Verification items for the finished model (mm, model axes). Face numbers are marked on the shaded views. Give positions to 0.01 mm unless a question says otherwise; leave off trailing zeros. Order: outer loops, then holes, each group sorted by start corner. A loop starts at its lowest first (then second) coordinate and runs counter-clockwise, first axis right, second up. Notation, with made-up numbers: (20.5, -19.75) - (58.5, -19.75) arc R16 ccw to (58.5, 6.25) - close; hole circle Ø4 at (65.25, 57). An arc over 180 degrees is marked (long way). Answer as a JSON object with one key per item and string values. Group by question number.
(1) Section check D-D (y = 30). Record the boundary of the cut face in (x, z) (1 decimal).
(2) Mould release check, pull along X, two halves, no side actions. Record for the marked faces 1, 2 and 3: +X half, -X half, draft (parallel to the pull), parting line (faces both ways), or undercut.
(3) Thickness scan on line 1 (X direction, y = -0.8, z = 0); line 2 (X direction, y = 35.2, z = 0); line 3 (Y direction, x = -7, z = 0.25). Record the ranges inside material, lowest first.
(4) Section check B-B (z = 0). Count the separate pieces of the cut face and the enclosed holes in it, then the cut area to 3 significant figures.
(5) Section check C-C (x = 0). Record the boundary of the cut face in (y, z).
(6) Depth check by flat-ended pin: pin 1 Ø1.1 at (x, z) = (0, 9) entering from -Y; pin 2 Ø0.5 at (x, y) = (12.5, -0.5) entering from +Z; pin 3 Ø0.5 at (x, y) = (-13.5, -0.5) entering from -Z. Enter the tip coordinate at first touch or a pass-through.
(7) Section check A-A (y = 6). Record the boundary of the cut face in (x, z) (1 decimal).
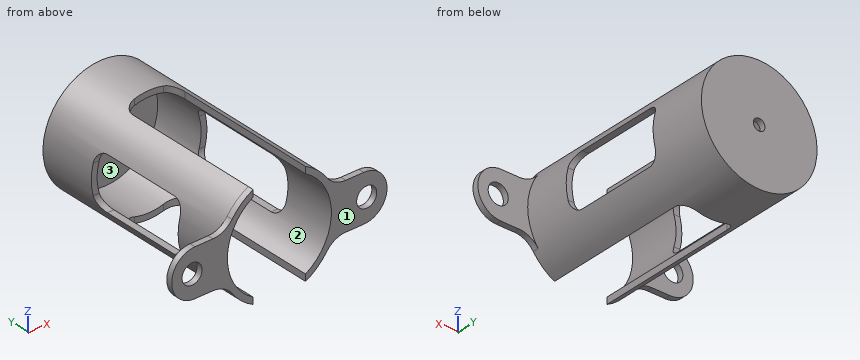
```python
from build123d import *

# Parameters (mm, degrees)
SKETCH2_R           = 9.9375
BOSS_EXTRUDE1_DEPTH = 35.384
SKETCH4_R           = 1
CUT_EXTRUDE2_DEPTH  = 39.072762817
BOSS_EXTRUDE2_START = 1
SKETCH11_R          = 8.9375
BOSS_EXTRUDE2_DEPTH = 1
SKETCH12_R          = 8.9375
CUT_EXTRUDE7_DEPTH  = 34.384
CUT_EXTRUDE8_START  = -1
CUT_EXTRUDE8_DEPTH  = 26.538
SKETCH14_W          = 9
SKETCH14_H          = 17.692
CUT_EXTRUDE9_DEPTH  = 61.852537846
FILLET3_R           = 2
FILLET4_R           = 4
CUT_EXTRUDE10_REACH = 43.146
SKETCH15_R          = 1.7272


# Read off the part's stored shape, not the designer's step: Cut-Extrude8
with BuildPart() as part:
    # Sketch2 → Boss-Extrude1 (new body)
    with BuildSketch(Plane(origin=(0, 0, 0), x_dir=(1, 0, 0), z_dir=(0, 1, 0))):
        with Locations(Location((0, 0, 0), (0, 0, 270))):
            Circle(SKETCH2_R)
    extrude(amount=BOSS_EXTRUDE1_DEPTH)

    # Sketch4 → Cut-Extrude2 (cut, through all)
    with BuildSketch(Plane(origin=(0, 35.384, 0), x_dir=(1, 0, 0), z_dir=(0, 1, 0))):
        with Locations(Location((0, 0, 0), (0, 0, 270))):
            Circle(SKETCH4_R)
    extrude(amount=-CUT_EXTRUDE2_DEPTH, mode=Mode.SUBTRACT)

    # Sketch11 → Boss-Extrude2 (add)
    with BuildSketch(Plane.XZ.offset(BOSS_EXTRUDE2_START)):
        with BuildLine():
            Line((9.096917404, 4), (18.5, 4))
            Line((18.5, 4), (18.5, -4))
            Line((18.5, -4), (9.096917404, -4))
            ThreePointArc((9.096917404, -4), (0, -9.9375), (-9.096917404, -4))
            Line((-9.096917404, -4), (-18.5, -4))
            Line((-18.5, -4), (-18.5, 4))
            Line((-18.5, 4), (-9.096917404, 4))
            ThreePointArc((-9.096917404, 4), (0, 9.9375), (9.096917404, 4))
        make_face()
        with Locations(Location((0, 0, 0), (0, 0, 270))):
            Circle(SKETCH11_R, mode=Mode.SUBTRACT)
    extrude(amount=-BOSS_EXTRUDE2_DEPTH)

    # Sketch12 → Cut-Extrude7 (cut)
    with BuildSketch(Plane.XZ):
        with Locations(Location((0, 0, 0), (0, 0, 270))):
            Circle(SKETCH12_R)
    extrude(amount=-CUT_EXTRUDE7_DEPTH, mode=Mode.SUBTRACT)

    # Cut-Extrude8 outline → Cut-Extrude8 (cut)
    with BuildSketch(Plane(origin=(0, 0, 0), x_dir=(1, 0, 0), z_dir=(0, 1, 0)).offset(CUT_EXTRUDE8_START)):
        with BuildLine():
            ThreePointArc((4.5, -7.721975541), (0, -8.9375), (-4.5, -7.721975541))
            Line((-4.5, -7.721975541), (-4.5, -8.860243013))
            ThreePointArc((-4.5, -8.860243013), (0, -9.9375), (4.5, -8.860243013))
            Line((4.5, -8.860243013), (4.5, -7.721975541))
        make_face()
        with BuildLine():
            Line((-4.5, 8.860243013), (-4.5, 7.721975541))
            ThreePointArc((-4.5, 7.721975541), (0, 8.9375), (4.5, 7.721975541))
            Line((4.5, 7.721975541), (4.5, 8.860243013))
            ThreePointArc((4.5, 8.860243013), (0, 9.9375), (-4.5, 8.860243013))
        make_face()
    extrude(amount=CUT_EXTRUDE8_DEPTH, mode=Mode.SUBTRACT)

    # Sketch14 → Cut-Extrude9 (cut, through all)
    with BuildSketch(Plane(origin=(30, 0, 0), x_dir=(0, 0, -1), z_dir=(1, 0, 0))):
        with Locations((0, 16.692)):
            Rectangle(SKETCH14_W, SKETCH14_H)
    extrude(amount=-CUT_EXTRUDE9_DEPTH, mode=Mode.SUBTRACT)

    # Fillet3
    fillet3_edges = [part.edges().sort_by_distance(p)[0] for p in [
        (4.5, 25.538, 8.291109277),
        (4.5, 25.538, -8.291109277),
        (-4.5, 25.538, -8.291109277),
        (-4.5, 25.538, 8.291109277),
        (8.291109277, 25.538, -4.5),
        (-8.291109277, 25.538, -4.5),
        (8.291109277, 7.846, -4.5),
        (-8.291109277, 7.846, -4.5),
        (-8.291109277, 7.846, 4.5),
        (8.291109277, 7.846, 4.5),
        (8.291109277, 25.538, 4.5),
        (-8.291109277, 25.538, 4.5),
    ]]
    fillet(fillet3_edges, radius=FILLET3_R)

    # Fillet4
    # the kernel refuses this fillet: 4 mm, written as the material it adds along each edge
    with BuildSketch(Plane(origin=(9.096917404, -1, -4), x_dir=(-0.4906341894667762, 0, -0.8713656477772574), z_dir=(0, 1, 0)), Plane(origin=(-9.096917404, -1, 4), x_dir=(0.49063418946677706, 0, 0.871365647777257), z_dir=(0, 1, 0))) as fillet4_piece_1:
        with BuildLine():
            CenterArc((2.349170519, -3.980589921), FILLET4_R, 95.646730554, 54.970995912)
            Line((-1.136292073, -2.018053163), (0, 0))
            ThreePointArc((0, 0), (0.977796106, -0.048221916), (1.955592212, 0))
        make_face()
    extrude(amount=1)
    with BuildSketch(Plane(origin=(9.096917404, -1, 4), x_dir=(-0.4906341894667768, 0, 0.8713656477772572), z_dir=(0, 1, 0)), Plane(origin=(-9.096917404, -1, -4), x_dir=(0.4906341894667772, 0, -0.8713656477772569), z_dir=(0, 1, 0))) as fillet4_piece_2:
        with BuildLine():
            CenterArc((2.349170519, 3.980589921), FILLET4_R, 209.382273534, 54.970995912)
            Line((-1.136292073, 2.018053163), (0, 0))
            ThreePointArc((0, 0), (0.977796106, 0.048221916), (1.955592212, 0))
        make_face()
    extrude(amount=1)
    # the kernel refuses this fillet: 4 mm, written as the material it takes off along each edge
    with BuildSketch(Plane(origin=(18.5, -11, -4), x_dir=(0, 0, 1), z_dir=(0, 1, 0)), Plane(origin=(18.5, -11, 4), x_dir=(-1, 0, 0), z_dir=(0, 1, 0))) as fillet4_2_piece_1:
        with BuildLine():
            CenterArc((FILLET4_R, -FILLET4_R), FILLET4_R, 90, 90)
            Line((0, -FILLET4_R), (0, 0))
            Line((0, 0), (FILLET4_R, 0))
        make_face()
    extrude(amount=21, mode=Mode.SUBTRACT)
    with BuildSketch(Plane(origin=(-18.5, -11, -4), x_dir=(0, 0, 1), z_dir=(0, 1, 0)), Plane(origin=(-18.5, -11, 4), x_dir=(1, 0, 0), z_dir=(0, 1, 0))) as fillet4_2_piece_2:
        with BuildLine():
            CenterArc((FILLET4_R, FILLET4_R), FILLET4_R, 180, 90)
            Line((0, FILLET4_R), (0, 0))
            Line((0, 0), (FILLET4_R, 0))
        make_face()
    extrude(amount=21, mode=Mode.SUBTRACT)

    # Sketch15 → Cut-Extrude10 (cut, up to next)
    with BuildSketch(Plane(origin=(0, 0, 0), x_dir=(1, 0, 0), z_dir=(0, 1, 0)), mode=Mode.PRIVATE) as cut_extrude10_sk1:
        with Locations(Location((-15, 0, 0), (0, 0, 270))):
            Circle(SKETCH15_R)
    cut_extrude10_tool1 = extrude(cut_extrude10_sk1.sketch, amount=-CUT_EXTRUDE10_REACH, mode=Mode.PRIVATE) & part.part
    # Sketch15 → Cut-Extrude10 (cut, up to next)
    with BuildSketch(Plane(origin=(0, 0, 0), x_dir=(1, 0, 0), z_dir=(0, 1, 0)), mode=Mode.PRIVATE) as cut_extrude10_sk2:
        with Locations(Location((15, 0, 0), (0, 0, 270))):
            Circle(SKETCH15_R)
    cut_extrude10_tool2 = extrude(cut_extrude10_sk2.sketch, amount=-CUT_EXTRUDE10_REACH, mode=Mode.PRIVATE) & part.part
    add(cut_extrude10_tool1.solids().sort_by_distance((-15, 0, 0))[0], mode=Mode.SUBTRACT)
    add(cut_extrude10_tool2.solids().sort_by_distance((15, 0, 0))[0], mode=Mode.SUBTRACT)


solid = part.part
```
Solutions:
{
 "1": {"outline": "circle Ø19.9 at (0, 0); hole circle Ø17.9 at (0, 0)"},
 "2": {"face 1": "draft", "face 2": "undercut", "face 3": "undercut"},
 "3": {"line 1": "x = -18.5 to -16.73, -13.27 to -8.94, 8.94 to 13.27, 16.73 to 18.5", "line 2": "x = -9.94 to -1, 1 to 9.94", "line 3": "y = 34.38 to 35.38"},
 "4": {"separate pieces": "6", "enclosed holes": "0", "area": "63.5 mm2"},
 "5": {"outline": "(25.54, -9.94) - (35.38, -9.94) - (35.38, -1) - (34.38, -1) - (34.38, -8.94) - (25.54, -8.94) - close; (25.54, 8.94) - (34.38, 8.94) - (34.38, 1) - (35.38, 1) - (35.38, 9.94) - (25.54, 9.94) - close"},
 "6": {"pin 1": "stops at y = 25.54", "pin 2": "stops at z = 4", "pin 3": "stops at z = -4"},
 "7": {"outline": "(-4.5, -8.9) - (-4.5, -7.7) arc R8.9 cw to (-4.5, 7.7) - (-4.5, 8.9) arc R9.9 ccw to start; (4.5, -8.9) arc R9.9 ccw to (4.5, 8.9) - (4.5, 7.7) arc R8.9 cw to (4.5, -7.7) - close"}
}
